from build123d import *

# Parameters (mm, degrees)
SKETCH1_R            = 75.925
BOSS_EXTRUDE1_DEPTH  = 2.5
SKETCH2_W            = 112.3
SKETCH2_H            = 40
CUT_EXTRUDE1_DEPTH   = 3.5
SKETCH10_R           = 75.925
SKETCH10_R_2         = 70.925
BOSS_EXTRUDE2_DEPTH  = 4
CUT_SWEEP3_PROFILE_R = 1.5


with BuildPart() as part:
    # Sketch1 → Boss-Extrude1 (new body)
    with BuildSketch(Plane(origin=(0, 0, 0), x_dir=(1, 0, 0), z_dir=(0, 1, 0))):
        Circle(SKETCH1_R)
    extrude(amount=BOSS_EXTRUDE1_DEPTH)

    # Sketch2 → Cut-Extrude1 (cut, through all)
    with BuildSketch(Plane(origin=(0, 2.5, 0), x_dir=(1, 0, 0), z_dir=(0, 1, 0))):
        with Locations((5, 0)):
            Rectangle(SKETCH2_W, SKETCH2_H)
    extrude(amount=-CUT_EXTRUDE1_DEPTH, mode=Mode.SUBTRACT)

    # Sketch10 → Boss-Extrude2 (add)
    with BuildSketch(Plane(origin=(0, 2.5, 0), x_dir=(1, 0, 0), z_dir=(0, 1, 0))):
        Circle(SKETCH10_R)
        Circle(SKETCH10_R_2, mode=Mode.SUBTRACT)
    extrude(amount=BOSS_EXTRUDE2_DEPTH)

    # Cut-Sweep3: sweep along a path in Sketch12
    with BuildLine(Plane(origin=(0, 6.5, 0), x_dir=(1, 0, 0), z_dir=(0, 1, 0))) as cut_sweep3_path:
        CenterArc((0, 0), 73.425, 0, 360)
    # Cut-Sweep3 profile (on start of the path) → Cut-Sweep3 (sweep, cut)
    with BuildSketch(Plane(origin=(73.425, 6.5, 0), x_dir=(-1, 0, 0), z_dir=(0, 0, -1))):
        Circle(CUT_SWEEP3_PROFILE_R)
    sweep(path=cut_sweep3_path.line, mode=Mode.SUBTRACT)


solid = part.part
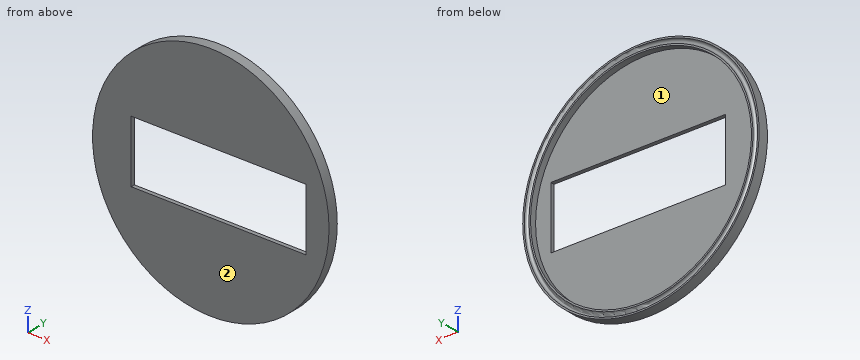
Verification items for the finished model (mm, model axes). Face numbers are marked on the shaded views. Coordinates: 2 decimals unless noted, no trailing zeros. Order: outer loops, then holes, each group sorted by start corner. A loop starts at its lowest first (then second) coordinate and runs counter-clockwise, first axis right, second up.
Item 1: Depth check by flat-ended pin: pin 1 (3 mm diameter, centred on x = -22.5, y = 3.5, fed in from +Z); pin 2 (2 mm diameter, centred on x = 3, y = 1, fed in from -Z); pin 3 (2 mm diameter, centred on x = 23, y = 1.5, fed in from +Z). Enter the tip coordinate at first touch or a pass-through.
Filled in:
pin 1: stops at z = 72.96
pin 2: stops at z = -75.9
pin 3: stops at z = 72.67
Item 2: Release check for a two-part mould opening along Z. For the marked faces 1 and 2 record: +Z half, -Z half, draft (parallel to the pull), parting line (faces both ways), or undercut.
Filled in:
face 1: undercut
face 2: draft
Item 3: Section check B-B, the plane z = 0. Enter the section's corners in (x, y) (3 decimals), then the cut area to 3 significant figures.
Filled in:
outline: (-75.925, 0) - (-51.15, 0) - (-51.15, 2.5) - (-70.925, 2.5) - (-70.925, 6.5) - (-71.925, 6.5) arc R1.5 cw to (-74.925, 6.5) - (-75.925, 6.5) - close; (61.15, 0) - (75.925, 0) - (75.925, 6.5) - (74.925, 6.5) arc R1.5 cw to (71.925, 6.5) - (70.925, 6.5) - (70.925, 2.5) - (61.15, 2.5) - close
area: 132 mm2
Item 4: Section check A-A, the plane x = 0. Enter the section's corners in (y, z) (3 decimals).
Filled in:
outline: (0, -75.925) - (6.5, -75.925) - (6.5, -74.925) arc R1.5 cw to (6.5, -71.925) - (6.5, -70.925) - (2.5, -70.925) - (2.5, -20) - (0, -20) - close; (0, 20) - (2.5, 20) - (2.5, 70.925) - (6.5, 70.925) - (6.5, 71.925) arc R1.5 cw to (6.5, 74.925) - (6.5, 75.925) - (0, 75.925) - close
Item 5: Material ranges on L1, parallel to Z at x = 0, y = 4.2 (3 decimals); L2, parallel to Z at x = 0, y = 5.5 (3 decimals), recorded low to high.
Filled in:
L1: z = -75.925 to -70.925, 70.925 to 75.925
L2: z = -75.925 to -74.543, -72.307 to -70.925, 70.925 to 72.307, 74.543 to 75.925
